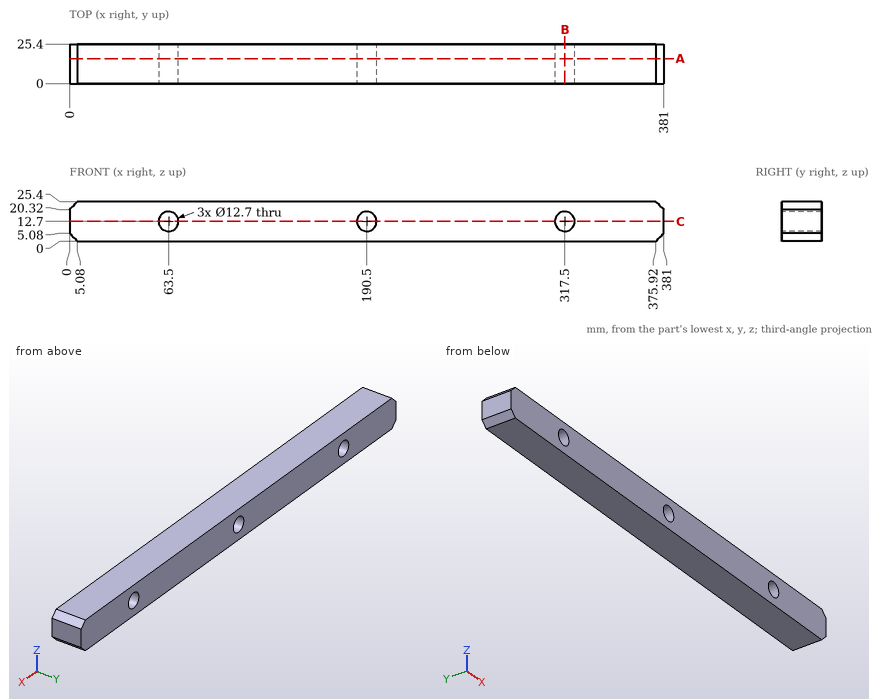
Answer from the drawing. Dimensions are ordinates in mm from the lowest x, y and z of the part. Coordinates: 2 decimals unless noted, no trailing zeros. Loops run counter-clockwise (first coordinate to the right, second up) from the corner with the lowest first, then second, coordinate; pieces in that order, holes last. Notation, with made-up numbers: (65, 56) -> (104, 56) arc R17 cw to (104, 87) -> close; hole circle Ø2 at (41.25, 43). An arc over 180 degrees is marked (long way). Answer as CSV lines item,"result".
Q1. The part is cut by section A-A on y = 16. Write down the section's boundary in (x, z), and give its area (3 significant figures).
Findings:
outline,"(0, 5.08) -> (5.08, 0) -> (375.92, 0) -> (381, 5.08) -> (381, 20.32) -> (375.92, 25.4) -> (5.08, 25.4) -> (0, 20.32) -> close; hole circle Ø12.7 at (63.5, 12.7); hole circle Ø12.7 at (190.5, 12.7); hole circle Ø12.7 at (317.5, 12.7)"
area,"9,250 mm²"
Q2. The part is cut by section C-C on z = 12.7. Write down the section's boundary in (x, y), and give its area (3 significant figures).
Findings:
outline,"(0, 0) -> (57.15, 0) -> (57.15, 25.4) -> (0, 25.4) -> close; (69.85, 0) -> (184.15, 0) -> (184.15, 25.4) -> (69.85, 25.4) -> close; (196.85, 0) -> (311.15, 0) -> (311.15, 25.4) -> (196.85, 25.4) -> close; (323.85, 0) -> (381, 0) -> (381, 25.4) -> (323.85, 25.4) -> close"
area,"8,710 mm²"
Q3. Find the intervals of material crossed by probe 1 along X at (y, z) = (21, 14); probe 2 along Z at (x, y) = (317.5, 6.5); probe 3 along X at (y, z) = (9.5, 13.75), in increasing order.
Findings:
probe 1,"x = 0 to 57.28, 69.72 to 184.28, 196.72 to 311.28, 323.72 to 381"
probe 2,"z = 0 to 6.35, 19.05 to 25.4"
probe 3,"x = 0 to 57.24, 69.76 to 184.24, 196.76 to 311.24, 323.76 to 381"
Q4. The part is cut by section B-B on x = 317.5. Write down the section's boundary in (y, z), and give its area (3 significant figures).
Findings:
outline,"(0, 0) -> (25.4, 0) -> (25.4, 6.35) -> (0, 6.35) -> close; (0, 19.05) -> (25.4, 19.05) -> (25.4, 25.4) -> (0, 25.4) -> close"
area,"323 mm²"
Q5. This flat-tipped pin is pushed along its axis until it touches: pin 1 (1 mm diameter, centred on x = 167.5, z = 12, fed in from -Y). Where does it stop, or does it pass through?
Findings:
pin 1,"stops at y = 0"
